Source: CAD feature listing. Evaluate the final solid. Frame: model axes, mm. A direction names the side the tool comes from. Coordinates: 2 decimals unless noted, no trailing zeros. Write each loop counter-clockwise with the first axis right and the second up, starting at its lowest first coordinate (ties: lowest second). Pieces come first, ordered by that corner, then holes. Notation, with made-up numbers: (77.5, 37) - (110.5, 37) arc R32 ccw to (110.5, 73) - close; hole circle Ø7 at (26, -40). An arc over 180 degrees is marked (long way). One line per question, with ' | ' between items.
from build123d import *

# Parameters (mm, degrees)
F0_W     = 100
F0_H     = 20
F1_DEPTH = 20
F3_DEPTH = 25
F4_W     = 58.4087243304
F4_H     = 10
F4_W_2   = 35
F4_H_2   = 8
F5_DEPTH = 25
F6_R     = 1.75
F7_DEPTH = 25
F8_R     = 3


with BuildPart() as f1:
    # F0 (on Top) → F1 (new body)
    with BuildSketch(Plane.XY):
        Rectangle(F0_W, F0_H)
    extrude(amount=F1_DEPTH)

    # F2 (on face) → F3 (cut)
    with BuildSketch(Plane.XZ.offset(10)):
        with BuildLine():
            ThreePointArc((-46.3747727085, 20), (-45.5257786585, 17.38335013), (-43.3, 19))
            ThreePointArc((-43.3, 19), (-43.38335013, 19.5257786585), (-43.6252272915, 20))
            Line((-43.6252272915, 20), (-46.3747727085, 20))
        make_face()
        with BuildLine():
            Line((0.3747727085, 20), (-2.3747727085, 20))
            ThreePointArc((-2.3747727085, 20), (-1.5257786585, 17.38335013), (0.7, 19))
            ThreePointArc((0.7, 19), (0.61664987, 19.5257786585), (0.3747727085, 20))
        make_face()
    extrude(amount=-F3_DEPTH, mode=Mode.SUBTRACT)

    # F4 (on face) → F5 (cut)
    with BuildSketch(Plane.XZ.offset(10)):
        Polygon((50, 20), (8.4087243304, 20), (8.4087243304, 10), (8.4087243304, 0), (50, 0), align=None)
        with Locations((-20.7956378348, 5)):
            Rectangle(F4_W, F4_H)
        with Locations((-23.2489995997, 16)):
            Rectangle(F4_W_2, F4_H_2)
    extrude(amount=-F5_DEPTH, mode=Mode.SUBTRACT)

    # F6 (on face) → F7 (cut)
    with BuildSketch(Plane(origin=(0, 0, 10), x_dir=(1, 0, 0), z_dir=(0, 0, -1))):
        with Locations((-35, 6)):
            Circle(F6_R)
        with Locations((5, 6)):
            Circle(F6_R)
    extrude(amount=-F7_DEPTH, mode=Mode.SUBTRACT)

    # F8
    f8_edges = [f1.edges().sort_by_distance(p)[0] for p in [
        (-50, -10, 15),
        (-50, 10, 15),
        (8.408724, 10, 15),
        (8.408724, -10, 15),
    ]]
    fillet(f8_edges, radius=F8_R)


solid = f1.part
Item 1: Mould query, pull axis X, two halves, no side actions, for faces 3 (the face through (-48, 0, 20)), 4 (the face through (-40.749, 0, 16)), 5 (the face through (-36.39, -4.94, 10.99)), 6 (the face through (7.51, -9.14, 14.93)). Classes: pulls with the +X half, pulls with the -X half, needs draft (parallel to the pull), parting line crosses it, or undercut.
Check sheet entries:
face 3: needs draft | face 4: undercut | face 5: undercut | face 6: pulls with the +X half
Item 2: Cut plane C-C on z = 16.5. Return loops of the section in (x, y), and give its area (3 significant figures).
Check sheet entries:
outline: (-50, -7) arc R3 ccw to (-47, -10) - (-40.75, -10) - (-40.75, 10) - (-47, 10) arc R3 ccw to (-50, 7) - close; (-5.75, -10) - (5.41, -10) arc R3 ccw to (8.41, -7) - (8.41, 7) arc R3 ccw to (5.41, 10) - (-5.75, 10) - close; hole circle Ø3.5 at (5, -6) | area: 451 mm²
Item 3: Cut plane D-D on y = 3. Return loops of the section in (x, z).
Check sheet entries:
outline: (-50, 10) - (8.41, 10) - (8.41, 20) - (0.37, 20) arc R1.7 cw (long way) to (-2.37, 20) - (-5.75, 20) - (-5.75, 12) - (-40.75, 12) - (-40.75, 20) - (-43.63, 20) arc R1.7 cw (long way) to (-46.37, 20) - (-50, 20) - close
Item 4: Pin query (flat end, axial travel): pin 1 Ø4.5 at (x, z) = (-45, 19) entering from -Y; pin 2 Ø3 at (x, y) = (-28, 3.5) entering from +Z. Return the tip coordinate at first contact, or that it passes through.
Check sheet entries:
pin 1: y = -10 | pin 2: z = 12
Item 5: Cut plane B-B on x = -35. Return loops of the section in (y, z), and give its area (3 significant figures).
Check sheet entries:
outline: (-10, 10) - (-7.75, 10) - (-7.75, 12) - (-10, 12) - close; (-4.25, 10) - (10, 10) - (10, 12) - (-4.25, 12) - close | area: 33.0 mm²
Item 6: Cut plane A-A on y = -6. Return loops of the section in (x, z).
Check sheet entries:
outline: (-50, 10) - (-36.75, 10) - (-36.75, 12) - (-40.75, 12) - (-40.75, 20) - (-43.63, 20) arc R1.7 cw (long way) to (-46.37, 20) - (-50, 20) - close; (-33.25, 10) - (3.25, 10) - (3.25, 20) - (0.37, 20) arc R1.7 cw (long way) to (-2.37, 20) - (-5.75, 20) - (-5.75, 12) - (-33.25, 12) - close; (6.75, 10) - (8.41, 10) - (8.41, 20) - (6.75, 20) - close
Item 7: Ray query, line 1 along X through (y, z) = (-6, 16.5); line 2 along X through (y, z) = (5.75, 19); line 3 along Y through (x, z) = (-35, 10.8). Return the intervals inside material, ascending. Write a range as [from, to].
Check sheet entries:
line 1: [-50, -40.75], [-5.75, 3.25], [6.75, 8.41] | line 2: [-50, -46.7], [-43.3, -40.75], [-5.75, -2.7], [0.7, 8.41] | line 3: [-10, -7.75], [-4.25, 10]
Item 8: Access query for faces 1 (the face through (-5.749, 0, 16)), 2 (the face through (-49.14, -9.1, 15.07)). Directions: +Z, -Z, +X, -X, +Y, -Y. A direction counts if a zero-diameter tool reaches every point of the face in a straight line with its end or side. Return the directions, or none.
Check sheet entries:
face 1: +Z, +Y, -Y | face 2: +Z, -Z, -X, -Y
